Check sheet for the modelled part. Datum: model origin and axes. Units: mm. A direction names the side the tool comes from. Give positions to 0.01 mm unless a question says otherwise; leave off trailing zeros. Write each loop counter-clockwise with the first axis right and the second up, starting at its lowest first coordinate (ties: lowest second). Pieces come first, ordered by that corner, then holes. Notation, with made-up numbers: (51, 44.5) -> (62, 44.5) arc R17 cw to (62, 48.5) -> close; hole circle Ø8 at (2.25, -1.5). An arc over 180 degrees is marked (long way). Use a Markdown table: item, result. Add a question column.
1. Cross-section at D-D (z = -0.25). Enter the section's corners in (x, y), then the cut area to 3 significant figures.
2. Set-up check for faces 4 (the flat face through (-3, -19, 5)), 5 (the cylindrical face through (21.791, -30.836, -0.07)): record each of +Z, -Z, +X, -X, +Y, -Y from which the full face is reachable in a straight line by a thin tool's end or side.
3. Cross-section at B-B (y = -41.5). Enter the section's corners in (x, z), then the cut area to 3 significant figures.
4. Scan lines: probe 1 along Y at (x, z) = (5.5, 2); probe 2 along Y at (x, z) = (-6.5, 1.25); probe 3 along Y at (x, z) = (15, -4). Record each from-to range of solid material in increasing order. Write a range as [from, to].
5. Cross-section at C-C (x = -10). Enter the section's corners in (y, z), then the cut area to 3 significant figures.
6. Cross-section at A-A (x = 0). Enter the section's corners in (y, z).
7. Gauge pin test, flat ends, axial feed: P1, Ø1, axis at y = -43.5, z = -3.5, coming from the +X side; P2, Ø12, axis at x = -27.5, y = -7.5, coming from the +Z side; P3, Ø4, axis at y = -48.5, z = -1.5, coming from the -X side; P4, Ø3, axis at y = -33.5, z = -2.5, coming from the +X side. Record the tip position at first contact, or that the pin passes through.
8. Release check for a two-part mould opening along Y. For faces 1 (the flat face through (-3, -19, -5)), 2 (the cylindrical face through (-30.41, -15.28, 0.07)), 3 (the flat face through (12.234, -38.372, 0.07)) record: released by +Y, released by -Y, zero draft, split by the parting line, or undercut.
from build123d import *

# Parameters (mm, degrees)
F0_R     = 7.5
F1_DEPTH = 5
F2_R     = 3
F5_D     = 5


with BuildPart() as f1:
    # F0 (on Top) → F1 (new body, symmetric)
    with BuildSketch(Plane.XY):
        with BuildLine():
            Line((-7.5, -40), (-7.5, -23.84848))
            ThreePointArc((-7.5, -23.84848), (20.155644, 14.790199), (-25, 0))
            ThreePointArc((-25, 0), (-30.562061, -15.466566), (-44.700474, -23.84848))
            ThreePointArc((-44.700474, -23.84848), (-31.474239, -30.881099), (-24.642584, -44.212248))
            ThreePointArc((-24.642584, -44.212248), (7.982755, -63.691256), (22.166723, -28.439879))
            Line((22.166723, -28.439879), (5.303301, -45.303301))
            ThreePointArc((5.303301, -45.303301), (-2.870126, -46.929096), (-7.5, -40))
        make_face()
        Circle(F0_R, mode=Mode.SUBTRACT)
    extrude(amount=F1_DEPTH, both=True)

    # F2
    f2_edges = [f1.edges().sort_by_distance(p)[0] for p in [
        (22.166723, -28.439879, 0),
        (-7.5, -23.84848, 0),
    ]]
    fillet(f2_edges, radius=F2_R)

    # F5 (through all)
    with Locations(Plane.XY):
        with Locations((-10, -10)):
            Hole(F5_D / 2)


solid = f1.part
Worked answers:
| question | item | result |
|---|---|---|
| 1 | outline | (-44.7, -23.85) arc R25 cw to (-24.64, -44.21) arc R25 ccw (long way) to (23.97, -32.9) arc R3 ccw to (18.97, -31.63) -> (5.3, -45.3) arc R7.5 cw to (-7.5, -40) -> (-7.5, -27.64) arc R3 cw to (-4.02, -24.68) arc R25 ccw (long way) to (-25, 0) arc R24.29 cw to start; hole circle Ø5 at (-10, -10); hole circle Ø15 at (0, 0) |
| 1 | area | 3,360 mm² |
| 2 | face 4 | +Z, +X, -X, +Y, -Y |
| 2 | face 5 | +Z, -Z |
| 3 | outline | (-25.26, -5) -> (-7.35, -5) -> (-7.35, 5) -> (-25.26, 5) -> close; (9.11, -5) -> (24.95, -5) -> (24.95, 5) -> (9.11, 5) -> close |
| 3 | area | 338 mm² |
| 4 | probe 1 | y = [-64.39, -45.11], [-24.39, -5.1], [5.1, 24.39] |
| 4 | probe 2 | y = [-64.14, -43.74], [-25.4, -3.74], [3.74, 24.14] |
| 4 | probe 3 | y = [-60, -35.61], [-20, 20] |
| 5 | outline | (-62.91, -5) -> (-12.5, -5) -> (-12.5, 5) -> (-62.91, 5) -> close; (-7.5, -5) -> (22.91, -5) -> (22.91, 5) -> (-7.5, 5) -> close |
| 5 | area | 808 mm² |
| 6 | outline | (-65, -5) -> (-47.5, -5) -> (-47.5, 5) -> (-65, 5) -> close; (-25, -5) -> (-7.5, -5) -> (-7.5, 5) -> (-25, 5) -> close; (7.5, -5) -> (25, -5) -> (25, 5) -> (7.5, 5) -> close |
| 7 | P1 | stops at x = 24.82 |
| 7 | P2 | stops at z = 5 |
| 7 | P3 | stops at x = -24.14 |
| 7 | P4 | stops at x = 24.49 |
| 8 | face 1 | zero draft |
| 8 | face 2 | released by +Y |
| 8 | face 3 | undercut |
